from build123d import *

# Parameters (mm, degrees)
F2_DEPTH  = 8
F3_DEPTH  = 8.001
F4_R      = 2.4
F5_DEPTH  = 8.001
F6_R      = 3.1
F7_DEPTH  = 0.8
F8_R      = 3.1
F9_DEPTH  = 0.8
F10_R     = 0.1
F11_R     = 0.1
F13_DEPTH = 3.1
F15_DEPTH = 3.1


with BuildPart() as f2:
    # F1 (on Top) → F2 (new body)
    with BuildSketch(Plane.XY):
        with BuildLine():
            ThreePointArc((3.6, 8), (0, 11.6), (-3.6, 8))
            Line((-3.6, 8), (-3.6, 0))
            ThreePointArc((-3.6, 0), (-2.5455844123, -2.5455844123), (0, -3.6))
            Line((0, -3.6), (24, -3.6))
            ThreePointArc((24, -3.6), (27.6, 0), (24, 3.6))
            Line((24, 3.6), (3.6, 3.6))
            Line((3.6, 3.6), (3.6, 8))
        make_face()
    extrude(amount=F2_DEPTH)

    # F0 (on Top) → F3 (cut, through all)
    with BuildSketch(Plane.XY):
        with BuildLine():
            Line((20.8, 2.8), (20, 2.8))
            Line((20, 2.8), (19.2, 2.8))
            ThreePointArc((19.2, 2.8), (18.8422291236, 2.5788854382), (18.88, 2.16))
            ThreePointArc((18.88, 2.16), (19.6, 0), (18.88, -2.16))
            ThreePointArc((18.88, -2.16), (18.8422291236, -2.5788854382), (19.2, -2.8))
            Line((19.2, -2.8), (20, -2.8))
            Line((20, -2.8), (20.8, -2.8))
            ThreePointArc((20.8, -2.8), (21.1577708764, -2.5788854382), (21.12, -2.16))
            ThreePointArc((21.12, -2.16), (20.8650842723, -1.7698314554), (20.6627106808, -1.35))
            ThreePointArc((20.6627106808, -1.35), (20.7018581261, -0.9763932023), (21.0335206052, -0.8))
            Line((21.0335206052, -0.8), (23.2, -0.8))
            Line((23.2, -0.8), (23.2, -2.2627416998))
            ThreePointArc((23.2, -2.2627416998), (24, -2.4), (24.8, -2.2627416998))
            Line((24.8, -2.2627416998), (24.8, -0.8))
            Line((24.8, -0.8), (26.2627416998, -0.8))
            ThreePointArc((26.2627416998, -0.8), (26.4, 0), (26.2627416998, 0.8))
            Line((26.2627416998, 0.8), (24.8, 0.8))
            Line((24.8, 0.8), (24.8, 2.2627416998))
            ThreePointArc((24.8, 2.2627416998), (24, 2.4), (23.2, 2.2627416998))
            Line((23.2, 2.2627416998), (23.2, 0.8))
            Line((23.2, 0.8), (21.0335206052, 0.8))
            ThreePointArc((21.0335206052, 0.8), (20.7018581261, 0.9763932023), (20.6627106808, 1.35))
            ThreePointArc((20.6627106808, 1.35), (20.8650842723, 1.7698314554), (21.12, 2.16))
            ThreePointArc((21.12, 2.16), (21.1577708764, 2.5788854382), (20.8, 2.8))
        make_face()
    extrude(amount=F3_DEPTH, mode=Mode.SUBTRACT)

    # F4 (on face) → F5 (cut, through all)
    with BuildSketch(Plane.XY):
        with Locations((16, 0)):
            Circle(F4_R)
        with Locations((8, 0)):
            Circle(F4_R)
        Circle(F4_R)
        with Locations((0, 8)):
            Circle(F4_R)
    extrude(amount=F5_DEPTH, mode=Mode.SUBTRACT)

    # F6 (on face) → F7 (cut)
    with BuildSketch(Plane.XY):
        with Locations((16, 0)):
            Circle(F6_R)
        with Locations((8, 0)):
            Circle(F6_R)
        Circle(F6_R)
        with Locations((0, 8)):
            Circle(F6_R)
    extrude(amount=F7_DEPTH, mode=Mode.SUBTRACT)

    # F8 (on face) → F9 (cut)
    with BuildSketch(Plane.XY.offset(8)):
        Circle(F8_R)
        with Locations((0, 8)):
            Circle(F8_R)
        with Locations((8, 0)):
            Circle(F8_R)
        with Locations((16, 0)):
            Circle(F8_R)
    extrude(amount=-F9_DEPTH, mode=Mode.SUBTRACT)

    # F10
    f10_edges = [f2.edges().sort_by_distance(p)[0] for p in [
        (0, 11.6, 8),
        (3.6, 5.8, 8),
        (13.8, 3.6, 8),
        (27.6, 0, 8),
        (12, -3.6, 8),
        (-2.545584, -2.545584, 8),
        (-3.6, 4, 8),
    ]]
    fillet(f10_edges, radius=F10_R)

    # F11
    f11_edges = [f2.edges().sort_by_distance(p)[0] for p in [
        (12, -3.6, 0),
        (27.6, 0, 0),
        (13.8, 3.6, 0),
        (3.6, 5.8, 0),
        (0, 11.6, 0),
        (-3.6, 4, 0),
        (-2.545584, -2.545584, 0),
    ]]
    fillet(f11_edges, radius=F11_R)

    # F12 (on face) → F13 (cut)
    with BuildSketch(Plane.XY):
        with BuildLine():
            Line((4, -2.8), (4.8, -2.8))
            ThreePointArc((4.8, -2.8), (5.1577708764, -2.5788854382), (5.12, -2.16))
            ThreePointArc((5.12, -2.16), (4.4, 0), (5.12, 2.16))
            ThreePointArc((5.12, 2.16), (5.1577708764, 2.5788854382), (4.8, 2.8))
            Line((4.8, 2.8), (4, 2.8))
            Line((4, 2.8), (3.2, 2.8))
            ThreePointArc((3.2, 2.8), (2.8422291236, 2.5788854382), (2.88, 2.16))
            ThreePointArc((2.88, 2.16), (3.6, 0), (2.88, -2.16))
            ThreePointArc((2.88, -2.16), (2.8422291236, -2.5788854382), (3.2, -2.8))
            Line((3.2, -2.8), (4, -2.8))
        make_face()
        with BuildLine():
            Line((2.8, 3.2), (2.8, 4))
            Line((2.8, 4), (2.8, 4.8))
            ThreePointArc((2.8, 4.8), (2.5788854382, 5.1577708764), (2.16, 5.12))
            ThreePointArc((2.16, 5.12), (1.1384199577, 4.584740127), (0, 4.4))
            ThreePointArc((0, 4.4), (-1.1384199577, 4.584740127), (-2.16, 5.12))
            ThreePointArc((-2.16, 5.12), (-2.5788854382, 5.1577708764), (-2.8, 4.8))
            Line((-2.8, 4.8), (-2.8, 4))
            Line((-2.8, 4), (-2.8, 3.2))
            ThreePointArc((-2.8, 3.2), (-2.5788854382, 2.8422291236), (-2.16, 2.88))
            ThreePointArc((-2.16, 2.88), (-1.1384199577, 3.415259873), (0, 3.6))
            ThreePointArc((0, 3.6), (1.1384199577, 3.415259873), (2.16, 2.88))
            ThreePointArc((2.16, 2.88), (2.5788854382, 2.8422291236), (2.8, 3.2))
        make_face()
        with BuildLine():
            ThreePointArc((10.88, -2.16), (10.8422291236, -2.5788854382), (11.2, -2.8))
            Line((11.2, -2.8), (12, -2.8))
            Line((12, -2.8), (12.8, -2.8))
            ThreePointArc((12.8, -2.8), (13.1577708764, -2.5788854382), (13.12, -2.16))
            ThreePointArc((13.12, -2.16), (12.4, 0), (13.12, 2.16))
            ThreePointArc((13.12, 2.16), (13.1577708764, 2.5788854382), (12.8, 2.8))
            Line((12.8, 2.8), (12, 2.8))
            Line((12, 2.8), (11.2, 2.8))
            ThreePointArc((11.2, 2.8), (10.8422291236, 2.5788854382), (10.88, 2.16))
            ThreePointArc((10.88, 2.16), (11.6, 0), (10.88, -2.16))
        make_face()
    extrude(amount=F13_DEPTH, mode=Mode.SUBTRACT)

    # F14 (on face) → F15 (cut)
    with BuildSketch(Plane.XY.offset(8)):
        with BuildLine():
            ThreePointArc((10.88, -2.16), (10.8422291236, -2.5788854382), (11.2, -2.8))
            Line((11.2, -2.8), (12, -2.8))
            Line((12, -2.8), (12.8, -2.8))
            ThreePointArc((12.8, -2.8), (13.1577708764, -2.5788854382), (13.12, -2.16))
            ThreePointArc((13.12, -2.16), (12.4, 0), (13.12, 2.16))
            ThreePointArc((13.12, 2.16), (13.1577708764, 2.5788854382), (12.8, 2.8))
            Line((12.8, 2.8), (12, 2.8))
            Line((12, 2.8), (11.2, 2.8))
            ThreePointArc((11.2, 2.8), (10.8422291236, 2.5788854382), (10.88, 2.16))
            ThreePointArc((10.88, 2.16), (11.6, 0), (10.88, -2.16))
        make_face()
        with BuildLine():
            Line((4, -2.8), (4.8, -2.8))
            ThreePointArc((4.8, -2.8), (5.1577708764, -2.5788854382), (5.12, -2.16))
            ThreePointArc((5.12, -2.16), (4.4, 0), (5.12, 2.16))
            ThreePointArc((5.12, 2.16), (5.1577708764, 2.5788854382), (4.8, 2.8))
            Line((4.8, 2.8), (4, 2.8))
            Line((4, 2.8), (3.2, 2.8))
            ThreePointArc((3.2, 2.8), (2.8422291236, 2.5788854382), (2.88, 2.16))
            ThreePointArc((2.88, 2.16), (3.6, 0), (2.88, -2.16))
            ThreePointArc((2.88, -2.16), (2.8422291236, -2.5788854382), (3.2, -2.8))
            Line((3.2, -2.8), (4, -2.8))
        make_face()
        with BuildLine():
            ThreePointArc((-2.16, 2.88), (-1.1384199577, 3.415259873), (0, 3.6))
            ThreePointArc((0, 3.6), (1.1384199577, 3.415259873), (2.16, 2.88))
            ThreePointArc((2.16, 2.88), (2.5788854382, 2.8422291236), (2.8, 3.2))
            Line((2.8, 3.2), (2.8, 4))
            Line((2.8, 4), (2.8, 4.8))
            ThreePointArc((2.8, 4.8), (2.5788854382, 5.1577708764), (2.16, 5.12))
            ThreePointArc((2.16, 5.12), (1.1384199577, 4.584740127), (0, 4.4))
            ThreePointArc((0, 4.4), (-1.1384199577, 4.584740127), (-2.16, 5.12))
            ThreePointArc((-2.16, 5.12), (-2.5788854382, 5.1577708764), (-2.8, 4.8))
            Line((-2.8, 4.8), (-2.8, 4))
            Line((-2.8, 4), (-2.8, 3.2))
            ThreePointArc((-2.8, 3.2), (-2.5788854382, 2.8422291236), (-2.16, 2.88))
        make_face()
    extrude(amount=-F15_DEPTH, mode=Mode.SUBTRACT)


solid = f2.part
Geometry check sheet. Reference: the model listing, model coordinates, mm. A direction names the side the tool comes from. Give positions to 0.01 mm unless a question says otherwise; leave off trailing zeros. Loops run counter-clockwise (first coordinate to the right, second up) from the corner with the lowest first, then second, coordinate; pieces in that order, holes last. Notation, with made-up numbers: M 43,-1 L 63,-1 A30 ccw 63,24 Z; hole C 2.5,82.5 d4. An arc over 180 degrees is marked long. Write each question's results on one line, items separated by ' | '.
1) Tool access check on faces 1 (the face through (4.9, 0.1, 7.6)), 2 (the face through (2.8, 4, 2)), 3 (the face through (26, 0.8, 4)). Record the directions out of +Z, -Z, +X, -X, +Y, -Y that give a thin tool (end or side, any length) a straight path to the whole face; none if there is none.
Answers follow:
face 1: +Z | face 2: -Z | face 3: +Z, -Z
2) Release check for a two-part mould opening along Y. For faces 4 (the face through (10.8, 1.8, 0)), 5 (the face through (20, 2.8, 4)) record: +Y half, -Y half, draft (parallel to the pull), parting line (faces both ways), or undercut.
Answers follow:
face 4: draft | face 5: undercut
3) Section check D-D, the plane x = 6. Record the boundary of the cut face in (y, z).
Answers follow:
outline: M -3.6,0.1 A0.1 ccw -3.5,0 L -2.37,0 L -2.37,0.8 L -1.33,0.8 L -1.33,7.2 L -2.37,7.2 L -2.37,8 L -3.5,8 A0.1 ccw -3.6,7.9 Z; M 1.33,0.8 L 2.37,0.8 L 2.37,0 L 3.5,0 A0.1 ccw 3.6,0.1 L 3.6,7.9 A0.1 ccw 3.5,8 L 2.37,8 L 2.37,7.2 L 1.33,7.2 Z
4) Section check C-C, the plane z = 3.5. Count the separate pieces of the cut face and the enclosed holes in it, plus the area to 3 significant figures.
Answers follow:
separate pieces: 1 | enclosed holes: 5 | area: 173 mm2
5) Section check A-A, the plane x = 16. Record the boundary of the cut face in (y, z).
Answers follow:
outline: M -3.6,0.1 A0.1 ccw -3.5,0 L -3.1,0 L -3.1,0.8 L -2.4,0.8 L -2.4,7.2 L -3.1,7.2 L -3.1,8 L -3.5,8 A0.1 ccw -3.6,7.9 Z; M 2.4,0.8 L 3.1,0.8 L 3.1,0 L 3.5,0 A0.1 ccw 3.6,0.1 L 3.6,7.9 A0.1 ccw 3.5,8 L 3.1,8 L 3.1,7.2 L 2.4,7.2 Z
6) Thickness scan on line 1 (Y direction, x = 8, z = 7.45); line 2 (Y direction, x = 22, z = 2); line 3 (Y direction, x = 19, z = 1). Record the ranges inside material, lowest first.
Answers follow:
line 1: -3.6 to -3.1, 3.1 to 3.6 | line 2: -3.6 to -0.8, 0.8 to 3.6 | line 3: -3.6 to -2.75, -1.99 to 1.99, 2.75 to 3.6
7) Gauge pin test, flat ends, axial feed: pin 1 (2.5 mm diameter, centred on x = 22.5, z = 2.5, fed in from +Y); pin 2 (3 mm diameter, centred on x = 17, y = 0, fed in from -Z); pin 3 (5.5 mm diameter, centred on x = 0, y = 0, fed in from +Z). Record the tip position at first contact, or that the pin passes through.
Answers follow:
pin 1: y = 3.6 | pin 2: z = 0.8 | pin 3: z = 7.2
8) Section check B-B, the plane y = 4. Record the boundary of the cut face in (x, z), plus the area to 3 significant figures.
Answers follow:
outline: M -3.6,0.1 A0.1 ccw -3.5,0 L -2.8,0 L -2.8,3.1 L 2.8,3.1 L 2.8,0 L 3.5,0 A0.1 ccw 3.6,0.1 L 3.6,7.9 A0.1 ccw 3.5,8 L 2.8,8 L 2.8,4.9 L -2.8,4.9 L -2.8,8 L -3.5,8 A0.1 ccw -3.6,7.9 Z | area: 22.9 mm2
